Build history of the part. All positions in model axes, mm. Face numbers are marked on the shaded views. A direction names the side the tool comes from. Round coordinates to 2 decimals unless told otherwise and drop trailing zeros. Order: outer loops, then holes, each group sorted by start corner. A loop starts at its lowest first (then second) coordinate and runs counter-clockwise, first axis right, second up. Notation, with made-up numbers: M -2,31 L 18,31 A21 cw 18,44 Z; hole C 1.25,-19 d6. An arc over 180 degrees is marked long. One line per item, written item: value. Start each with the question number.
Item 1: Pin check, flat tips, straight feed: pin 1 (3 mm diameter, centred on x = 0, y = 1, fed in from +Z); pin 2 (1.5 mm diameter, centred on x = -1, z = -23.5, fed in from -Y); pin 3 (3 mm diameter, centred on x = -1.5, z = -29, fed in from +Y); pin 4 (4 mm diameter, centred on y = -2.5, z = -35.5, fed in from -X). Stop position of each tip, or through.
Item 2: Tool access for the marked faces 1 and 2: list every direction of +Z, -Z, +X, -X, +Y, -Y with a clear straight run to the whole face (end or side of a thin tool).
Item 3: Band-saw the part on B-B, the plane z = -26.5. Write the cut outline in (x, y).
Item 4: Probe L1, parallel to Z at x = -1.25, y = -2; L2, parallel to Z at x = -0.25, y = 1.25; L3, parallel to X at y = 1, z = -26. List the from-to ranges inside material, lowest first.
Item 5: Band-saw the part on A-A, the plane x = 0. Write the cut outline in (y, z), then the cut area to 3 significant figures.
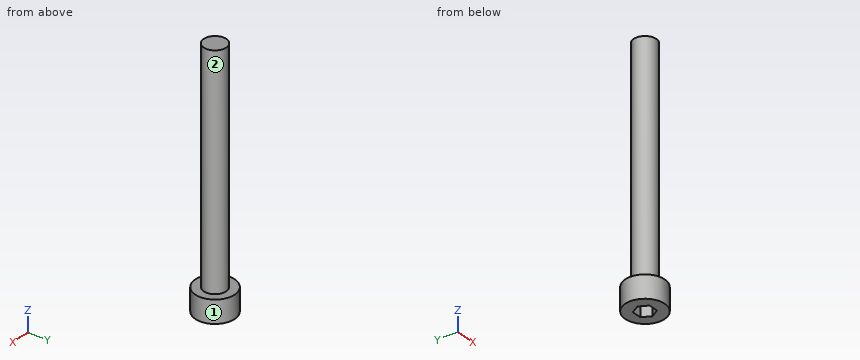
```python
from build123d import *

# Parameters (mm, degrees)
CUT_EXTRUDE1_DEPTH = 3


with BuildPart() as part:
    # Sketch1 → Revolve1 (revolve)
    with BuildSketch(Plane(origin=(0, 0, 0), x_dir=(1, 0, 0), z_dir=(0, 1, 0)), mode=Mode.PRIVATE) as revolve1_sk:
        Polygon((0, 0), (2, 0), (2, 40), (3.5, 40), (3.5, 44), (0, 44), align=None)
    revolve(revolve1_sk.sketch.rotate(Axis((0, 0, -44), (0, 0, 1)), 180), axis=Axis((0, 0, -44), (0, 0, 1)))

    # Sketch2 → Cut-Extrude1 (cut)
    with BuildSketch(Plane(origin=(0, 0, -44), x_dir=(-1, 0, 0), z_dir=(0, 0, -1))):
        Polygon((-0.866025404, -1.5), (0.866025404, -1.5), (1.732050808, 0), (0.866025404, 1.5), (-0.866025404, 1.5), (-1.732050808, 0), align=None)
    extrude(amount=-CUT_EXTRUDE1_DEPTH, mode=Mode.SUBTRACT)


solid = part.part
```
Output:
1. pin 1: stops at z = 0
1. pin 2: stops at y = -1.98
1. pin 3: stops at y = 2
1. pin 4: stops at x = -1.94
2. face 1: +Z, -Z
2. face 2: +Z
3. outline: C 0,0 d4
4. L1: z = -44 to -40
4. L2: z = -41 to 0
4. L3: x = -1.73 to 1.73
5. outline: M -3.5,-44 L -1.5,-44 L -1.5,-41 L 1.5,-41 L 1.5,-44 L 3.5,-44 L 3.5,-40 L 2,-40 L 2,0 L -2,0 L -2,-40 L -3.5,-40 Z
5. area: 179 mm²
